Verification items for the finished model (mm, model axes). Face numbers are marked on the shaded views. A direction names the side the tool comes from. Give positions to 0.01 mm unless a question says otherwise; leave off trailing zeros. Loops run counter-clockwise (first coordinate to the right, second up) from the corner with the lowest first, then second, coordinate; pieces in that order, holes last. Notation, with made-up numbers: (-9, 71) -> (36, 71) arc R8 cw to (36, 85) -> close; hole circle Ø7 at (-18.5, 28.5). An arc over 180 degrees is marked (long way). Answer in a Markdown table with one row per item. Add a question column.
Q1. Section check C-C on x = 0. Enter the section's corners in (y, z), and give its area (3 significant figures).
Q2. Section check D-D on x = -94. Enter the section's corners in (y, z).
Q3. Material ranges on probe 1 along Y at (x, z) = (-114, 31); probe 2 along X at (y, z) = (20, 89.5); probe 3 along X at (y, z) = (-17, 110), recorded low to high.
Q4. Set-up check for the marked faces 1, 2 and 3: record each of +Z, -Z, +X, -X, +Y, -Y from which the full face is reachable in a straight line by a thin tool's end or side.
Q5. Gauge pin test, flat ends, axial feed: P1, Ø2, axis at x = 118, z = 52.5, coming from the -Y side; P2, Ø6, axis at x = 93, z = 101.5, coming from the +Y side; P3, Ø1.5, axis at x = 91.5, y = 3.5, coming from the +Z side. Record the tip position at first contact, or that the pin passes through.
Q6. Section check A-A on y = 0. Enter the section's corners in (x, z), and give its area (3 significant figures).
Q7. Section check B-B on z = 122.5. Enter the section's corners in (x, y).
Q8. Release check for a two-part mould opening along X. For the marked faces 4, 5 and 6 record: pulls with the +X half, pulls with the -X half, needs draft (parallel to the pull), parting line crosses it, or undercut.
```python
from build123d import *

# Parameters (mm, degrees)
F0_W     = 304.8
F0_H     = 152.4
F0_R     = 25.4
F1_DEPTH = 152.4
F3_DEPTH = 101.6
F4_DEPTH = 177.801


with BuildPart() as f1:
    # F0 (on Top) → F1 (new body)
    with BuildSketch(Plane.XY):
        Rectangle(F0_W, F0_H)
        with Locations((-114.3, 0)):
            Circle(F0_R, mode=Mode.SUBTRACT)
        with Locations((114.3, 0)):
            Circle(F0_R, mode=Mode.SUBTRACT)
    extrude(amount=F1_DEPTH)

    # F2 (on Front) → F3 (join, symmetric)
    with BuildSketch(Plane.XZ):
        with BuildLine():
            Line((63.5, 152.4), (38.1, 152.4))
            ThreePointArc((38.1, 152.4), (0, 114.3), (-38.1, 152.4))
            Line((-38.1, 152.4), (-63.5, 152.4))
            ThreePointArc((-63.5, 152.4), (0, 88.9), (63.5, 152.4))
        make_face()
    extrude(amount=F3_DEPTH, both=True)

    # F4 (cut, through all): a face of the model
    f4_faces = [f1.faces().sort_by_distance(p)[0] for p in [
        (0, -76.2, 136.2298577819),
    ]]
    extrude(f4_faces, amount=-F4_DEPTH, mode=Mode.SUBTRACT)


solid = f1.part
```
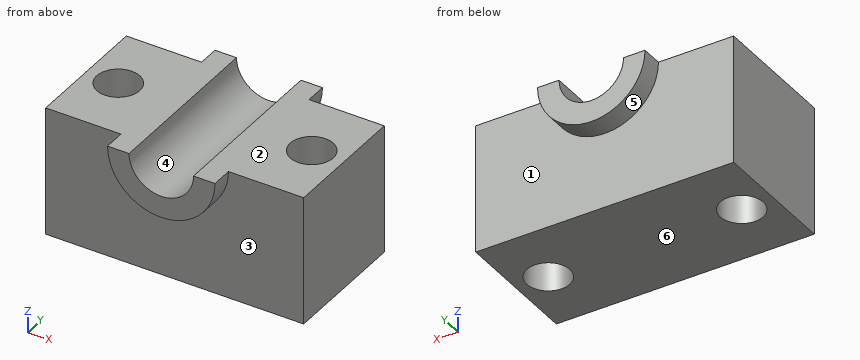
Taken from the geometry:
| question | item | result |
|---|---|---|
| 1 | outline | (-101.6, 88.9) -> (-76.2, 88.9) -> (-76.2, 0) -> (76.2, 0) -> (76.2, 88.9) -> (101.6, 88.9) -> (101.6, 114.3) -> (-101.6, 114.3) -> close |
| 1 | area | 18,700 mm² |
| 2 | outline | (-76.2, 0) -> (-15.27, 0) -> (-15.27, 152.4) -> (-76.2, 152.4) -> close; (15.27, 0) -> (76.2, 0) -> (76.2, 152.4) -> (15.27, 152.4) -> close |
| 3 | probe 1 | y = -76.2 to -25.4, 25.4 to 76.2 |
| 3 | probe 2 | x = -152.4 to -129.96, -98.64 to 98.64, 129.96 to 152.4 |
| 3 | probe 3 | x = -152.4 to -133.17, -95.43 to 95.43, 133.17 to 152.4 |
| 4 | face 1 | -Z, +Y |
| 4 | face 2 | +Z, +X, -X, +Y, -Y |
| 4 | face 3 | -Z, -Y |
| 5 | P1 | stops at y = -76.2 |
| 5 | P2 | stops at y = 76.2 |
| 5 | P3 | passes through |
| 6 | outline | (-152.4, 0) -> (-139.7, 0) -> (-139.7, 152.4) -> (-152.4, 152.4) -> close; (-88.9, 0) -> (88.9, 0) -> (88.9, 152.4) -> (38.1, 152.4) arc R38.1 cw to (-38.1, 152.4) -> (-88.9, 152.4) -> close; (139.7, 0) -> (152.4, 0) -> (152.4, 152.4) -> (139.7, 152.4) -> close |
| 6 | area | 28,700 mm² |
| 7 | outline | (-152.4, -76.2) -> (-56.02, -76.2) -> (-56.02, -101.6) -> (-23.61, -101.6) -> (-23.61, 101.6) -> (-56.02, 101.6) -> (-56.02, 76.2) -> (-152.4, 76.2) -> close; (23.61, -101.6) -> (56.02, -101.6) -> (56.02, -76.2) -> (152.4, -76.2) -> (152.4, 76.2) -> (56.02, 76.2) -> (56.02, 101.6) -> (23.61, 101.6) -> close; hole circle Ø50.8 at (-114.3, 0); hole circle Ø50.8 at (114.3, 0) |
| 8 | face 4 | undercut |
| 8 | face 5 | parting line crosses it |
| 8 | face 6 | needs draft |
